Geometry: final body of the model. Coordinates: model frame, mm. A direction names the side the tool comes from. Give positions to 0.01 mm unless a question says otherwise; leave off trailing zeros. Write each loop counter-clockwise with the first axis right and the second up, starting at its lowest first coordinate (ties: lowest second). Pieces come first, ordered by that corner, then holes.
from build123d import *

# Parameters (mm, degrees)
SKETCH1_W           = 16
SKETCH1_H           = 30
BOSS_EXTRUDE1_DEPTH = 8
SKETCH2_W           = 5.5
SKETCH2_H           = 30
BOSS_EXTRUDE2_DEPTH = 4.5
CHAMFER1_SIZE       = 2
SKETCH6_R           = 2.25
BOSS_EXTRUDE3_DEPTH = 6
FILLET6_R           = 3
CUT_EXTRUDE1_START  = -3
SKETCH7_W           = 16
SKETCH7_H           = 6.1
CUT_EXTRUDE1_DEPTH  = 2.8
CUT_EXTRUDE2_DEPTH  = 5
SKETCH9_W           = 4.5
SKETCH9_H           = 10.5
CUT_EXTRUDE3_DEPTH  = 1
SKETCH10_R          = 5
CUT_EXTRUDE4_DEPTH  = 2
FILLET7_R           = 3


with BuildPart() as part:
    # Sketch1 → Boss-Extrude1 (new body)
    with BuildSketch(Plane(origin=(0, 0, 0), x_dir=(0, 0, -1), z_dir=(1, 0, 0))):
        with Locations((-40.846556001, 12.91146402)):
            Rectangle(SKETCH1_W, SKETCH1_H)
    extrude(amount=BOSS_EXTRUDE1_DEPTH)

    # Sketch2 → Boss-Extrude2 (add)
    with BuildSketch(Plane.ZY):
        with Locations((40.846556001, 12.91146402)):
            Rectangle(SKETCH2_W, SKETCH2_H)
    extrude(amount=BOSS_EXTRUDE2_DEPTH)

    # Chamfer1
    chamfer1_edges = [part.edges().sort_by_distance(p)[0] for p in [
        (-4.5, -2.08853598, 40.846556001),
        (-4.5, 27.91146402, 40.846556001),
    ]]
    chamfer(chamfer1_edges, length=CHAMFER1_SIZE)

    # Sketch6 → Boss-Extrude3 (add)
    with BuildSketch(Plane.XZ.offset(2.08853598)):
        with BuildLine():
            Line((8, 48.846556001), (16, 48.846556001))
            ThreePointArc((16, 48.846556001), (24, 40.846556001), (16, 32.846556001))
            Line((16, 32.846556001), (8, 32.846556001))
            Line((8, 32.846556001), (8, 48.846556001))
        make_face()
        with Locations(Location((16, 40.846556001, 0), (0, 0, 270))):
            Circle(SKETCH6_R, mode=Mode.SUBTRACT)
    extrude(amount=-BOSS_EXTRUDE3_DEPTH)

    # Fillet6
    fillet6_edges = [part.edges().sort_by_distance(p)[0] for p in [
        (8, 3.91146402, 40.846556001),
    ]]
    fillet(fillet6_edges, radius=FILLET6_R)

    # Sketch7 → Cut-Extrude1 (cut)
    with BuildSketch(Plane(origin=(8, 0, 0), x_dir=(0, 0, -1), z_dir=(1, 0, 0)).offset(CUT_EXTRUDE1_START)):
        with Locations((-40.846556001, 20.91146402)):
            Rectangle(SKETCH7_W, SKETCH7_H)
        with Locations((-40.846556001, 10.41146402)):
            Rectangle(SKETCH7_W, SKETCH7_H)
    extrude(amount=-CUT_EXTRUDE1_DEPTH, mode=Mode.SUBTRACT)

    # Sketch8 → Cut-Extrude2 (cut)
    with BuildSketch(Plane(origin=(8, 0, 0), x_dir=(0, 0, -1), z_dir=(1, 0, 0))):
        with BuildLine():
            Line((-44.346556001, 22.76146402), (-37.346556001, 22.76146402))
            ThreePointArc((-37.346556001, 22.76146402), (-35.496556001, 20.91146402), (-37.346556001, 19.06146402))
            Line((-37.346556001, 19.06146402), (-44.346556001, 19.06146402))
            ThreePointArc((-44.346556001, 19.06146402), (-46.196556001, 20.91146402), (-44.346556001, 22.76146402))
        make_face()
        with BuildLine():
            Line((-44.346556001, 12.26146402), (-37.346556001, 12.26146402))
            ThreePointArc((-37.346556001, 12.26146402), (-35.496556001, 10.41146402), (-37.346556001, 8.56146402))
            Line((-37.346556001, 8.56146402), (-44.346556001, 8.56146402))
            ThreePointArc((-44.346556001, 8.56146402), (-46.196556001, 10.41146402), (-44.346556001, 12.26146402))
        make_face()
    extrude(amount=-CUT_EXTRUDE2_DEPTH, mode=Mode.SUBTRACT)

    # Sketch9 → Cut-Extrude3 (cut)
    with BuildSketch(Plane(origin=(8, 0, 0), x_dir=(0, 0, -1), z_dir=(1, 0, 0))):
        with Locations((-35.096556001, 15.66146402)):
            Rectangle(SKETCH9_W, SKETCH9_H)
    extrude(amount=-CUT_EXTRUDE3_DEPTH, mode=Mode.SUBTRACT)

    # Sketch10 → Cut-Extrude4 (cut)
    with BuildSketch(Plane(origin=(0, 3.91146402, 0), x_dir=(1, 0, 0), z_dir=(0, 1, 0))):
        with Locations(Location((16, -40.846556001, 0), (0, 0, 270))):
            Circle(SKETCH10_R)
    extrude(amount=-CUT_EXTRUDE4_DEPTH, mode=Mode.SUBTRACT)

    # Fillet7
    fillet7_edges = [part.edges().sort_by_distance(p)[0] for p in [
        (4, 27.91146402, 32.846556001),
        (4, 27.91146402, 48.846556001),
    ]]
    fillet(fillet7_edges, radius=FILLET7_R)


solid = part.part
Q1. Section C-C on y = 25.5. Output: boundary loops of the cut face in (x, z), plus the area to 3 significant figures.
Filled sheet:
outline: (-4.5, 38.1) - (0, 38.1) - (0, 32.9) - (8, 32.9) - (8, 48.79) - (0, 48.79) - (0, 43.6) - (-4.5, 43.6) - close
area: 152 mm2
Q2. Pin query (flat end, axial travel): P1, Ø6.5, axis at y = 21.5, z = 42.5, coming from the +X side; P2, Ø3.5, axis at x = 16, z = 40.85, coming from the -Y side; P3, Ø5, axis at x = 0, z = 46, coming from the +Y side; P4, Ø6.5, axis at x = 15, z = 37, coming from the +Y side. Return the tip coordinate at first contact, or that it passes through.
Filled sheet:
P1: stops at x = 8
P2: passes through
P3: stops at y = 27.91
P4: stops at y = 3.91
Q3. Section D-D on x = 11.75. Output: boundary loops of the cut face in (y, z), plus the area to 3 significant figures.
Filled sheet:
outline: (-2.09, 32.85) - (3.91, 32.85) - (3.91, 38.21) - (1.91, 38.21) - (1.91, 43.48) - (3.91, 43.48) - (3.91, 48.85) - (-2.09, 48.85) - close
area: 85.5 mm2
Q4. Section A-A on x = 16.75. Output: boundary loops of the cut face in (y, z), plus the area to 3 significant figures.
Filled sheet:
outline: (-2.09, 32.88) - (3.91, 32.88) - (3.91, 35.9) - (1.91, 35.9) - (1.91, 38.73) - (-2.09, 38.73) - close; (-2.09, 42.97) - (1.91, 42.97) - (1.91, 45.79) - (3.91, 45.79) - (3.91, 48.81) - (-2.09, 48.81) - close
area: 58.8 mm2
Q5. Access query for faces 1 (the cylindrical face through (14.085, 2.925, 45.465)), 2 (the flat face through (5, 12.5, 41)), 3 (the flat face through (0, 13, 46)), 4 (the flat face through (-2, 13, 38.097)). Directions: +Z, -Z, +X, -X, +Y, -Y. A direction counts if a zero-diameter tool reaches every point of the face in a straight line with its end or side. Return the directions, or none.
Filled sheet:
face 1: +Y
face 2: +Z, -Z
face 3: +Z, -X, +Y, -Y
face 4: -Z, -X, +Y, -Y
Q6. Pull-direction query (Z, two-part tool) for faces 5 (the cylindrical face through (6.2, 9.8, 35.6)), 6 (the flat face through (6, 8, 32.847)), 7 (the flat face through (-4.5, 13, 41)); classes: released by +Z, released by -Z, zero draft, split by the parting line, or undercut.
Filled sheet:
face 5: undercut
face 6: released by -Z
face 7: zero draft
Q7. Ray query, line 1 along Y through (x, z) = (3.5, 37.5); line 2 along Y through (x, z) = (6.25, 40.25); line 3 along X through (y, z) = (8.5, 46). Return the intervals inside material, ascending.
Filled sheet:
line 1: y = -2.09 to 7.36, 13.46 to 17.86, 23.96 to 27.91
line 2: y = -2.09 to 8.56, 12.26 to 19.06, 22.76 to 27.91
line 3: x = 0 to 2.2, 5 to 8
